Source: CAD feature listing. Evaluate the final solid. Frame: model axes, mm. Face numbers are marked on the shaded views. A direction names the side the tool comes from. Coordinates: 2 decimals unless noted, no trailing zeros. Write each loop counter-clockwise with the first axis right and the second up, starting at its lowest first coordinate (ties: lowest second). Pieces come first, ordered by that corner, then holes. Notation, with made-up numbers: (15, -13) -> (28, -13) arc R16 ccw to (28, 12) -> close; hole circle Ø11 at (17.25, 42). An arc over 180 degrees is marked (long way). One line per item, written item: value. Start each with the question number.
1. Section query A-A, the plane z = 0. Output: boundary loops of the cut face in (x, y).
2. First-contact query: P1, Ø4.5, axis at x = -40.9, z = -13.29, coming from the -Y side; P2, Ø2.5, axis at x = 25.27, z = 34.79, coming from the -Y side; P3, Ø1.2, axis at x = -40, y = 24, coming from the +Z side; P4, Ø1, axis at y = 14.5, z = -14, coming from the +X side. Flat tips, straight axial feed; report the tip coordinate or a pass-through.
3. Access query for the marked faces 4, 5 and 6. Directions: +Z, -Z, +X, -X, +Y, -Y. A direction counts if a zero-diameter tool reaches every point of the face in a straight line with its end or side. Return the directions, or none.
4. Line query: line 1 (Z direction, x = -23.5, y = 6); line 2 (Y direction, x = 5, z = 26); line 3 (Z direction, x = -44.5, y = 19). Output: solid intervals per line, ascending.
5. Section query B-B, the plane y = 20. State how many separate pieces and enclosed holes the cut face has, and give its area (3 significant figures).
6. Section query D-D, the plane x = 35.5. Output: boundary loops of the cut face in (y, z).
7. Section query C-C, the plane z = -43. Output: boundary loops of the cut face in (x, y), and give its area (3 significant figures).
8. Mould query, pull axis Z, two halves, no side actions, for the marked faces 1, 2 and 3. Classes: released by +Z, released by -Z, zero draft, split by the parting line, or undercut.
Autodesk Inventor part; units mm, degrees
ref_plane "РабПлоскость2" through (-36.8954, 36, 0) normal (0, 0, -1) x (-1, 0, 0)
ref_plane "YZ Plane" through (0, 0, 0) normal (1, 0, 0) x (0, 1, 0)
ref_plane "XZ Plane" through (0, 0, 0) normal (0, 1, 0) x (-1, 0, 0)
sketch "Эскиз12" plane through (0, 0, 0) normal (0, 1, 0) x (-1, 0, 0)
  line L0 (114.5, 15) -> (114.5, 11.5)
  line L1 (114.5, 11.5) -> (114.5, -11.5)
  line L2 (114.5, -11.5) -> (114.5, -15)
  line L3 (114.5, -15) -> (108.5, -20.1)
  line L4 (108.5, -20.1) -> (55.4, -20.1)
  line L5 (55.4, -20.1) -> (49.4, -15)
  line L6 (49.4, -15) -> (49.4, 15)
  line L7 (49.4, 15) -> (55.4, 20.1)
  line L8 (55.4, 20.1) -> (108.5, 20.1)
  line L9 (108.5, 20.1) -> (114.5, 15)
  arc A0 (-1.6711, 9.8594) -> (-9.8594, 1.6711) centre (0, 0) ccw
  arc A1 (1.6711, 9.8594) -> (-1.6711, 9.8594) centre (0, 8) ccw
  arc A2 (9.8594, 1.6711) -> (1.6711, 9.8594) centre (0, 0) ccw
  arc A3 (9.8594, -1.6711) -> (9.8594, 1.6711) centre (8, 0) ccw
  arc A4 (1.6711, -9.8594) -> (9.8594, -1.6711) centre (0, 0) ccw
  arc A5 (-1.6711, -9.8594) -> (1.6711, -9.8594) centre (0, -8) ccw
  arc A6 (-9.8594, -1.6711) -> (-1.6711, -9.8594) centre (0, 0) ccw
  arc A7 (-9.8594, 1.6711) -> (-9.8594, -1.6711) centre (-8, 0) ccw
  circle A8 centre (0, 43) radius 2
  circle A9 centre (-25.2748, 34.7877) radius 2
  circle A10 centre (-40.8954, 13.2877) radius 2
  circle A11 centre (-40.8954, -13.2877) radius 2
  circle A12 centre (-25.2748, -34.7877) radius 2
  circle A13 centre (0, -43) radius 2
  circle A14 centre (25.2748, -34.7877) radius 2
  circle A15 centre (40.8954, -13.2877) radius 2
  circle A16 centre (40.8954, 13.2877) radius 2
  circle A17 centre (25.2748, 34.7877) radius 2
  arc A18 (38.3107, 32.1293) -> (38.3107, -32.1293) centre (0, 0) ccw
  arc A19 (97.8335, -24.9059) -> (38.3107, -32.1293) centre (85.2244, -169.8586) ccw
  arc A20 (97.8335, -24.9059) -> (97.8335, 24.9059) centre (100, 0) ccw
  arc A21 (38.3107, 32.1293) -> (97.8335, 24.9059) centre (85.2244, 169.8586) ccw
  circle A22 centre (52.2, 11) radius 1.025
  circle A23 centre (52.2, -11) radius 1.025
  circle A24 centre (60, -17.3) radius 1.025
  circle A25 centre (60, 17.3) radius 1.025
  line L10 (55, -11.5) -> (55, 11.5)
  arc A26 (58, 14.5) -> (55, 11.5) centre (58, 11.5) ccw
  line L11 (58, 14.5) -> (111.5, 14.5)
  arc A27 (55, -11.5) -> (58, -14.5) centre (58, -11.5) ccw
  line L12 (111.5, -14.5) -> (58, -14.5)
  arc A28 (111.5, -14.5) -> (114.5, -11.5) centre (111.5, -11.5) ccw
  arc A29 (114.5, 11.5) -> (111.5, 14.5) centre (111.5, 11.5) ccw
  line L13 (40.8954, 13.2877) -> (40.8954, -13.2877)
  line L14 (36.8954, 18.5) -> (44.8954, 18.5)
  line L15 (44.8954, 18.5) -> (44.8954, -18.5)
  line L16 (44.8954, -18.5) -> (36.8954, -18.5)
  line L17 (36.8954, -18.5) -> (36.8954, 18.5)
  line L18 (36.8954, 18.5) -> (44.8954, -18.5) construction
  line L19 (44.8954, 18.5) -> (36.8954, -18.5) construction
  line L20 (44.8954, -18.5) -> (44.8954, -30.0593)
  line L21 (55.4, -20.1) -> (55.4, -27.448)
  line L22 (55.4, 20.1) -> (55.4, 27.448)
  line L23 (44.8954, 18.5) -> (44.8954, 30.0593)
  point P0 (40.8954, 0)
  dimension "d45" = 8
  dimension "d46" = 37
extrude "Выдавливание9" add sketch "Эскиз12" along normal blind 5 contours L7 L6 L5 L21 A19 L20 L15 L23 A21 L22 | L23 L14 L17 L16 L20 A19 A18 A21 | L15 L16 L17 L14
sketch "Эскиз13" plane through (0, 5, 0) normal (0, 1, 0) x (1, 0, 0)
  line L0 (-114.5, -15) -> (-114.5, -11.5)
  line L1 (-114.5, -11.5) -> (-114.5, 11.5)
  line L2 (-114.5, 11.5) -> (-114.5, 15)
  line L3 (-114.5, 15) -> (-108.5, 20.1)
  line L4 (-108.5, 20.1) -> (-55.4, 20.1)
  line L5 (-55.4, 20.1) -> (-49.4, 15)
  line L6 (-49.4, 15) -> (-49.4, -15)
  line L7 (-49.4, -15) -> (-55.4, -20.1)
  line L8 (-55.4, -20.1) -> (-108.5, -20.1)
  line L9 (-108.5, -20.1) -> (-114.5, -15)
  arc A0 (1.6711, -9.8594) -> (9.8594, -1.6711) centre (0, 0) ccw
  arc A1 (-1.6711, -9.8594) -> (1.6711, -9.8594) centre (0, -8) ccw
  arc A2 (-9.8594, -1.6711) -> (-1.6711, -9.8594) centre (0, 0) ccw
  arc A3 (-9.8594, 1.6711) -> (-9.8594, -1.6711) centre (-8, 0) ccw
  arc A4 (-1.6711, 9.8594) -> (-9.8594, 1.6711) centre (0, 0) ccw
  arc A5 (1.6711, 9.8594) -> (-1.6711, 9.8594) centre (0, 8) ccw
  arc A6 (9.8594, 1.6711) -> (1.6711, 9.8594) centre (0, 0) ccw
  arc A7 (9.8594, -1.6711) -> (9.8594, 1.6711) centre (8, 0) ccw
  circle A8 centre (0, -43) radius 2
  circle A9 centre (25.2748, -34.7877) radius 2
  circle A10 centre (40.8954, -13.2877) radius 2
  circle A11 centre (40.8954, 13.2877) radius 2
  circle A12 centre (25.2748, 34.7877) radius 2
  circle A13 centre (0, 43) radius 2
  circle A14 centre (-25.2748, 34.7877) radius 2
  circle A15 centre (-40.8954, 13.2877) radius 2
  circle A16 centre (-40.8954, -13.2877) radius 2
  circle A17 centre (-25.2748, -34.7877) radius 2
  arc A18 (-38.3107, -32.1293) -> (-38.3107, 32.1293) centre (0, 0) ccw
  arc A19 (-97.8335, 24.9059) -> (-38.3107, 32.1293) centre (-85.2244, 169.8586) ccw
  arc A20 (-97.8335, 24.9059) -> (-97.8335, -24.9059) centre (-100, 0) ccw
  arc A21 (-38.3107, -32.1293) -> (-97.8335, -24.9059) centre (-85.2244, -169.8586) ccw
  circle A22 centre (-52.2, -11) radius 1.025
  circle A23 centre (-52.2, 11) radius 1.025
  circle A24 centre (-60, 17.3) radius 1.025
  circle A25 centre (-60, -17.3) radius 1.025
  line L10 (-55, 11.5) -> (-55, -11.5)
  arc A26 (-58, -14.5) -> (-55, -11.5) centre (-58, -11.5) ccw
  line L11 (-58, -14.5) -> (-111.5, -14.5)
  arc A27 (-55, 11.5) -> (-58, 14.5) centre (-58, 11.5) ccw
  line L12 (-111.5, 14.5) -> (-58, 14.5)
  arc A28 (-111.5, 14.5) -> (-114.5, 11.5) centre (-111.5, 11.5) ccw
  arc A29 (-114.5, -11.5) -> (-111.5, -14.5) centre (-111.5, -11.5) ccw
  line L13 (-40.8954, -13.2877) -> (-40.8954, 13.2877)
  line L14 (-36.8954, -18.5) -> (-44.8954, -18.5)
  line L15 (-44.8954, -18.5) -> (-44.8954, 18.5)
  line L16 (-44.8954, 18.5) -> (-36.8954, 18.5)
  line L17 (-36.8954, 18.5) -> (-36.8954, -18.5)
  line L18 (-36.8954, -18.5) -> (-44.8954, 18.5) construction
  line L19 (-44.8954, -18.5) -> (-36.8954, 18.5) construction
  line L20 (-44.8954, 18.5) -> (-44.8954, 30.0593)
  line L21 (-55.4, 20.1) -> (-55.4, 27.448)
  line L22 (-55.4, -20.1) -> (-55.4, -27.448)
  line L23 (-44.8954, -18.5) -> (-44.8954, -30.0593)
  point P0 (0, 0)
  point P1 (-40.8954, 0)
  dimension "d49" = 8
  dimension "d50" = 37
extrude "Выдавливание10" add sketch "Эскиз13" along normal blind 31 contours L7 L6 L5 L21 A19 L20 L15 L23 A21 L22 | L15 L16 L17 L14
sketch "Эскиз14" plane through (-36.8954, 5, 18.5) normal (1, 0, 0) x (0, 0, -1)
  line L0 (3.2123, 0) -> (3.2123, 31)
  line L1 (7.2123, 0) -> (7.2123, 31)
  line L2 (29.7877, 0) -> (29.7877, 31)
  line L3 (33.7877, 0) -> (33.7877, 31)
  line L4 (3.2123, 19.2083) -> (7.2123, 19.2083)
  line L5 (1.5123, 17.2083) -> (8.9123, 17.2083)
  line L6 (8.9123, 17.2083) -> (8.9123, 21.2083)
  line L7 (8.9123, 21.2083) -> (1.5123, 21.2083)
  line L8 (1.5123, 21.2083) -> (1.5123, 17.2083)
  line L9 (1.5123, 17.2083) -> (8.9123, 21.2083) construction
  line L10 (8.9123, 17.2083) -> (1.5123, 21.2083) construction
  line L11 (29.7877, 19.2083) -> (33.7877, 19.2083)
  line L12 (28.0877, 17.2083) -> (35.4877, 17.2083)
  line L13 (35.4877, 17.2083) -> (35.4877, 21.2083)
  line L14 (35.4877, 21.2083) -> (28.0877, 21.2083)
  line L15 (28.0877, 21.2083) -> (28.0877, 17.2083)
  line L16 (28.0877, 17.2083) -> (35.4877, 21.2083) construction
  line L17 (35.4877, 17.2083) -> (28.0877, 21.2083) construction
  point P0 (5.2123, 19.2083)
  point P1 (31.7877, 19.2083)
  dimension "d53" = 7.4
  dimension "d54" = 4
  dimension "d55" = 7.4
  dimension "d56" = 4
extrude "Выдавливание11" cut sketch "Эскиз14" against normal blind 8
sketch "Эскиз16" plane through (0, 5, 0) normal (0, 1, 0) x (1, 0, 0)
  line L0 (0, -18.5) -> (-11.559, -18.5)
  line L1 (-11.559, -18.5) -> (-11.559, -30.059)
  line L2 (-11.559, -30.059) -> (0, -30.059)
  line L3 (0, -30.059) -> (0, -18.5)
  point P0 (0, 0)
  point P1 (-5.7795, -24.2795)
  dimension "d60" = 11.559
  dimension "d61" = 11.559
loft "Лофт1" add profiles "Эскиз16" section 2 edges at (-44.8954, 20.5, 18.5) (-44.8954, 36, 24.2797) (-44.8954, 20.5, 30.0593) (-44.8954, 5, 24.2797)
ref_plane "РабПлоскость2" through (-36.8954, 36, 0) normal (0, 0, -1) x (-1, 0, 0)
mirror "Зеркальное отражение2" about plane through (-36.8954, 36, 0) normal (0, 0, -1) of "Лофт1"
sketch "Эскиз17" plane through (0, 36, 0) normal (0, 1, 0) x (1, 0, 0)
  circle A0 centre (-40.8954, -13.2877) radius 2
  circle A1 centre (-40.8954, 13.2877) radius 2
  line L0 (-36.8954, -18.5) -> (-36.8954, 18.5)
  line L1 (-36.8954, 18.5) -> (-44.8954, 18.5)
  line L2 (-44.8954, 18.5) -> (-44.8954, 30.0593)
  arc A2 (-55.4, 27.448) -> (-44.8954, 30.0593) centre (-85.2244, 169.8586) ccw
  line L3 (-55.4, 27.448) -> (-55.4, 20.1)
  line L4 (-55.4, 20.1) -> (-49.4, 15)
  line L5 (-49.4, 15) -> (-49.4, -15)
  line L6 (-49.4, -15) -> (-55.4, -20.1)
  line L7 (-55.4, -20.1) -> (-55.4, -27.448)
  arc A3 (-44.8954, -30.0593) -> (-55.4, -27.448) centre (-85.2244, -169.8586) ccw
  line L8 (-44.8954, -30.0593) -> (-44.8954, -18.5)
  line L9 (-44.8954, -18.5) -> (-36.8954, -18.5)
  point P0 (0, 0)
properties part number "000.302 - Кожух" material "Пластик АБС"
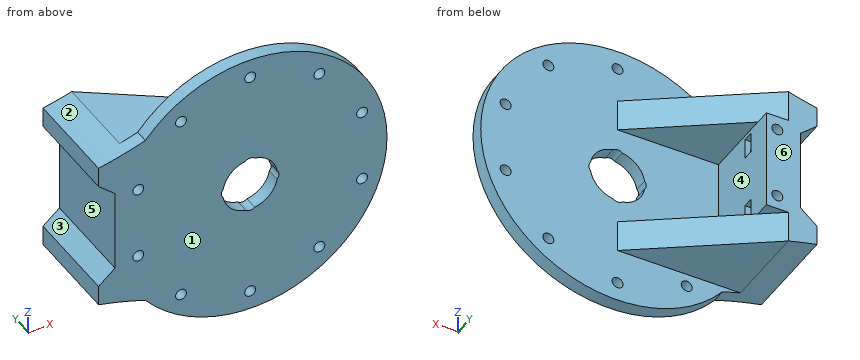
Computed values:
1. outline: (-49.4, 0) -> (-10.5, 0) -> (-10.5, 5) -> (-36.9, 5) -> (-36.9, 36) -> (-49.4, 36) -> close; (10.5, 0) -> (50, 0) -> (50, 5) -> (10.5, 5) -> close
2. P1: stops at y = 0
2. P2: passes through
2. P3: stops at z = 30.06
2. P4: stops at x = -36.9
3. face 4: +X, +Y
3. face 5: -X, +Y, -Y
3. face 6: +Z, -Z, +X, -X, +Y
4. line 1: z = -30.06 to -18.5, 18.5 to 30.06
4. line 2: y = 0 to 5
4. line 3: z = -30.06 to 30.06
5. separate pieces: 1
5. enclosed holes: 2
5. area: 1,200 mm²
6. outline: (0, -35.21) -> (5, -35.21) -> (5, 35.21) -> (0, 35.21) -> close
7. outline: (-25.51, 0) -> (-2, 0) -> (-2, 5) -> (-25.51, 5) -> close; (2, 0) -> (25.51, 0) -> (25.51, 5) -> (2, 5) -> close
7. area: 235 mm²
8. face 1: zero draft
8. face 2: released by +Z
8. face 3: undercut
